CAD build for the part. Positions are in the model's coordinates, mm. A direction names the side the tool comes from. Round coordinates to 2 decimals unless told otherwise and drop trailing zeros. Loops run counter-clockwise (first coordinate to the right, second up) from the corner with the lowest first, then second, coordinate; pieces in that order, holes last.
from build123d import *

# Parameters (mm, degrees)
SKETCH2_W             = 54.022158158
SKETCH2_H             = 36.022158158
SKETCH2_W_2           = 46.5
SKETCH2_H_2           = 28.5
BOSS_EXTRUDE1_DEPTH   = 34.036
SKETCH11_R            = 1.049999932
CUT_EXTRUDE1_DEPTH    = 74.310563675
BOSS_EXTRUDE3_DEPTH   = 6
BOSS_EXTRUDE3_2_DEPTH = 6
SKETCH19_W            = 8
SKETCH19_H            = 46.439396398
SKETCH19_W_2          = 24.86121623
SKETCH19_H_2          = 8
SKETCH19_W_3          = 6
SKETCH19_H_3          = 20
SKETCH19_W_4          = 20
SKETCH19_H_4          = 6
BOSS_EXTRUDE10_DEPTH  = 16
FILLET6_R             = 16
FILLET7_R             = 2
SKETCH21_R            = 1.7
CUT_EXTRUDE2_DEPTH    = 1.761079079
CUT_EXTRUDE3_START    = -1.761079079
SKETCH22_R            = 1.7
CUT_EXTRUDE3_DEPTH    = 1.761079079


with BuildPart() as part:
    # Sketch2 → Boss-Extrude1 (new body)
    with BuildSketch(Plane(origin=(0, 0, 0), x_dir=(1, 0, 0), z_dir=(0, 1, 0))):
        with Locations((27.011079079, -18.011079079)):
            Rectangle(SKETCH2_W, SKETCH2_H)
        with Locations((27.011079079, -18.011079079)):
            Rectangle(SKETCH2_W_2, SKETCH2_H_2, mode=Mode.SUBTRACT)
    extrude(amount=-BOSS_EXTRUDE1_DEPTH)

    # Sketch11 → Cut-Extrude1 (cut, through all)
    with BuildSketch(Plane(origin=(0, 0, 0), x_dir=(-1, 0, 0), z_dir=(0, 0, -1))):
        with Locations((-19.011079079, -11)):
            Circle(SKETCH11_R)
        with Locations((-19.011079079, -23)):
            Circle(SKETCH11_R)
        with Locations((-43.01107908, -11)):
            Circle(SKETCH11_R)
        with Locations((-43.011079079, -23)):
            Circle(SKETCH11_R)
    extrude(amount=-CUT_EXTRUDE1_DEPTH, mode=Mode.SUBTRACT)



with BuildPart() as body_2:
    # Sketch12 → Boss-Extrude3 (new body)
    with BuildSketch(Plane(origin=(0, 0, 0), x_dir=(1, 0, 0), z_dir=(0, 1, 0))):
        Polygon((0, -82.461554556), (-15, -82.461554556), (-21, -82.461554556), (-21, -62.461554556), (-15, -62.461554556), (0, -62.461554556), (8, -62.461554556), (8, -82.461554556), align=None)
    extrude(amount=BOSS_EXTRUDE3_DEPTH)


with BuildPart() as body_3:
    # Sketch12 → Boss-Extrude3 2 (new body)
    with BuildSketch(Plane(origin=(0, 0, 0), x_dir=(1, 0, 0), z_dir=(0, 1, 0))):
        Polygon((58.883374388, -8), (58.883374388, 0), (58.883374388, 15), (58.883374388, 21), (78.883374388, 21), (78.883374388, 15), (78.883374388, 0), (78.883374388, -8), align=None)
    extrude(amount=BOSS_EXTRUDE3_2_DEPTH)


with BuildPart() as part_1:
    add(part.part)

    add(body_2.part)  # Boss-Extrude10 merges body 2

    add(body_3.part)  # Boss-Extrude10 merges body 3
    # Sketch19 → Boss-Extrude10 (add)
    with BuildSketch(Plane(origin=(0, 0, 0), x_dir=(-1, 0, 0), z_dir=(0, 1, 0))):
        with Locations((-4, 59.241856357)):
            Rectangle(SKETCH19_W, SKETCH19_H)
        with Locations((-66.452766273, 4)):
            Rectangle(SKETCH19_W_2, SKETCH19_H_2)
        with Locations((18, 72.461554556)):
            Rectangle(SKETCH19_W_3, SKETCH19_H_3)
        with Locations((-68.883374388, -18)):
            Rectangle(SKETCH19_W_4, SKETCH19_H_4)
    extrude(amount=-BOSS_EXTRUDE10_DEPTH)

    # Fillet6
    fillet6_edges = [part_1.edges().sort_by_distance(p)[0] for p in [
        (78.883374388, -16, 4),
        (4, -16, 82.461554556),
    ]]
    fillet(fillet6_edges, radius=FILLET6_R)

    # Fillet7
    fillet7_edges = [part_1.edges().sort_by_distance(p)[0] for p in [
        (-21, -16, 72.461554556),
        (-15, -16, 72.461554556),
        (68.883374388, -16, -21),
        (68.883374388, -16, -15),
        (78.883374388, 3, 8),
        (54.022158158, -34.036, 18.011079079),
        (74.197082887, -11.313708499, 8),
        (8, 3, 82.461554556),
        (8, -16, 51.241856357),
        (8, -11.313708499, 77.775263055),
        (27.011079079, -34.036, 0),
        (0, -34.036, 18.011079079),
        (8, -8, 36.022158158),
        (4, -16, 36.022158158),
        (4, 0, 62.461554556),
        (-21, -5, 62.461554556),
        (-21, -5, 82.461554556),
        (8, 6, 72.461554556),
        (-6.5, 6, 62.461554556),
        (-21, 6, 72.461554556),
        (-6.5, 6, 82.461554556),
        (54.022158158, -17.018, 36.022158158),
        (58.452766273, -16, 8),
        (54.022158158, -16, 4),
        (54.022158158, -8, 8),
        (27.011079079, -34.036, 36.022158158),
        (78.883374388, -5, -21),
        (58.883374388, 0, 4),
        (58.883374388, -5, -21),
        (68.883374388, 6, 8),
        (78.883374388, 6, -6.5),
        (68.883374388, 6, -21),
        (58.883374388, 6, -6.5),
    ]]
    fillet(fillet7_edges, radius=FILLET7_R)

    # Sketch21 → Cut-Extrude2 (cut)
    with BuildSketch(Plane.XY.offset(36.022158158)):
        with Locations((19.011079079, -11)):
            Circle(SKETCH21_R)
        with Locations((43.01107908, -11)):
            Circle(SKETCH21_R)
        with Locations((19.011079079, -23)):
            Circle(SKETCH21_R)
        with Locations((43.011079079, -23)):
            Circle(SKETCH21_R)
    extrude(amount=-CUT_EXTRUDE2_DEPTH, mode=Mode.SUBTRACT)

    # Sketch22 → Cut-Extrude3 (cut)
    with BuildSketch(Plane(origin=(0, 0, 0), x_dir=(-1, 0, 0), z_dir=(0, 0, -1)).offset(CUT_EXTRUDE3_START)):
        with Locations(Location((-43.01107908, -11, 0), (0, 0, 180))):
            Circle(SKETCH22_R)
        with Locations(Location((-43.011079079, -23, 0), (0, 0, 180))):
            Circle(SKETCH22_R)
        with Locations(Location((-19.011079079, -11, 0), (0, 0, 180))):
            Circle(SKETCH22_R)
        with Locations(Location((-19.011079079, -23, 0), (0, 0, 180))):
            Circle(SKETCH22_R)
    extrude(amount=CUT_EXTRUDE3_DEPTH, mode=Mode.SUBTRACT)


solid = part_1.part
Item 1: Wall check: L1, parallel to X at y = -8, z = 73.5; L2, parallel to Z at x = 39, y = -26.5; L3, parallel to X at y = -29.5, z = 13. Give the ranges that are in metal, low to high.
Verdict:
L1: x = -21 to -15, 0 to 8
L2: z = 0 to 3.76, 32.26 to 36.02
L3: x = 0 to 3.76, 50.26 to 54.02
Item 2: Cut at C-C (y = -2). State how many separate pieces and enclosed holes the cut face has, plus the area to 3 significant figures.
Verdict:
separate pieces: 3
enclosed holes: 1
area: 1,420 mm2
Item 3: 3-axis set-ups, long thin cutter, end or side, ignore diameter. For faces 4 (the flat face through (54.022, -16, 21)), 5 (the cylindrical face through (17.313, -10.925, 35.154)), 6 (the flat face through (42, -10, 1.761)), 7 (the flat face through (50.261, -17, 18)): which of +Z, -Z, +X, -X, +Y, -Y reach the whole face in a straight line?
Verdict:
face 4: +Z, +X, -Y
face 5: +Z
face 6: -Z
face 7: +Y, -Y
Item 4: Cut at B-B (x = 23). List the corners of the cut face in (y, z), plus the area to 3 significant figures.
Verdict:
outline: (-34.04, 2) arc R2 ccw to (-32.04, 0) - (0, 0) - (0, 3.76) - (-34.04, 3.76) - close; (-34.04, 32.26) - (0, 32.26) - (0, 36.02) - (-32.04, 36.02) arc R2 ccw to (-34.04, 34.02) - close
area: 254 mm2
Item 5: Mould opens along X. For faces 1 (the flat face through (-21, -5, 73)), 2 (the flat face through (3, -16, 52)), 3 (the cylindrical face through (44.633, -11.511, 0.893)) say: released by +X, released by -X, zero draft, split by the parting line, or undercut.
Verdict:
face 1: released by -X
face 2: zero draft
face 3: undercut
Item 6: Flat gauge pins, fed straight in: P1, Ø2.5, axis at x = 43.01, y = -23, coming from the -Z side; P2, Ø16.5, axis at x = -6, z = 71, coming from the -Y side; P3, Ø3.5, axis at x = 43.5, y = -11, coming from the +Z side. Where does each tip first touch, or does it go through?
Verdict:
P1: stops at z = 1.76
P2: stops at y = -16
P3: stops at z = 36.02
Item 7: Cut at A-A (y = -26.5). List the corners of the cut face in (x, z), plus the area to 3 significant figures.
Verdict:
outline: (0, 0) - (54.02, 0) - (54.02, 34.02) arc R2 ccw to (52.02, 36.02) - (0, 36.02) - close; hole (3.76, 3.76) - (50.26, 3.76) - (50.26, 32.26) - (3.76, 32.26) - close
area: 620 mm2
